```python
from build123d import *

# Parameters (mm, degrees)
SKETCH1_W                = 20
SKETCH1_H                = 80
BOSS_EXTRUDE1_DEPTH      = 5
BOSS_EXTRUDE2_DEPTH      = 10
BOSS_EXTRUDE2_DEPTH_BACK = 5
SKETCH2_W                = 20
SKETCH2_H                = 10.2
SKETCH3_W                = 20
SKETCH3_H                = 4.2
CUT_EXTRUDE1_DEPTH       = 10
BOSS_EXTRUDE3_DEPTH      = 194.158928137


with BuildPart() as part:
    # Sketch1 → Boss-Extrude1 (new body)
    with BuildSketch(Plane(origin=(0, 0, 0), x_dir=(1, 0, 0), z_dir=(0, 1, 0))):
        with Locations((10, 40)):
            Rectangle(SKETCH1_W, SKETCH1_H)
    extrude(amount=BOSS_EXTRUDE1_DEPTH)

    # Sketch2 → Boss-Extrude2 (add, two sides: drawn at the far end of the back side and taken through both)
    with BuildSketch(Plane.XZ.offset(-BOSS_EXTRUDE2_DEPTH_BACK)):
        with Locations((10, 5.1)):
            Rectangle(SKETCH2_W, SKETCH2_H)
    extrude(amount=BOSS_EXTRUDE2_DEPTH + BOSS_EXTRUDE2_DEPTH_BACK)

    # Sketch3 → Cut-Extrude1 (cut)
    with BuildSketch(Plane.XZ.offset(10)):
        with Locations((10, 5.1)):
            Rectangle(SKETCH3_W, SKETCH3_H)
    extrude(amount=-CUT_EXTRUDE1_DEPTH, mode=Mode.SUBTRACT)

    # Sketch5 → Boss-Extrude3 (add)
    with BuildSketch(Plane.ZY):
        Polygon((3, 0), (7.2, 0), (7.2, 5), (-80, 5), (-80, 0), (0, 0), (0, -10), (3, -10), align=None)
        Polygon((7.2, -10), (10.2, -10), (10.2, 5), (7.2, 5), (7.2, 0), align=None)
    extrude(amount=BOSS_EXTRUDE3_DEPTH)


solid = part.part
```
Geometry: final body of the model. Coordinates: model frame, mm. A direction names the side the tool comes from. Coordinates: 2 decimals unless noted, no trailing zeros. Write each loop counter-clockwise with the first axis right and the second up, starting at its lowest first coordinate (ties: lowest second). Pieces come first, ordered by that corner, then holes. Notation, with made-up numbers: M -23,-37.75 L -18,-37.75 A33 cw -18,1.25 Z; hole C -16,27 d1. An arc over 180 degrees is marked long. Answer as CSV lines item,"result". Start each with the question number.
Q1. Cut plane C-C on z = -67.5. Return the cut outline in (x, y).
Q2. Pin query (flat end, axial travel): P1, Ø5, axis at x = -136, y = -7, coming from the -Z side; P2, Ø5, axis at x = -148, z = -22, coming from the -Y side. Return the tip coordinate at first contact, or that it passes through.
Q3. Mould query, pull axis Z, two halves, no side actions, for faces 4 (the flat face through (20, 1, -28)), 5 (the flat face through (-86, -5, 0)), 6 (the flat face through (-86, -5, 7.2)). Classes: released by +Z, released by -Z, zero draft, split by the parting line, or undercut.
Q4. Line query: line 1 (Z direction, x = -131, y = -1); line 2 (Y direction, x = -11.5, z = -22). Output: solid intervals per line, ascending. Write a range as from..to.
Q5. Reachability of faces 1 (the flat face through (-194.159, 1, -28)), 2 (the flat face through (-86, 0, -41)), 3 (the flat face through (-86, 0, 5)) from +Z, -Z, +X, -X, +Y, -Y: full face, straight path, thin tool, end or side. Return the list, or none.
Q6. Cut plane A-A on y = -2.5. Return the cut outline in (x, z).
Q7. Cut plane B-B on x = -75. Return the cut outline in (y, z).
Findings below:
1,outline,"M -194.16,0 L 20,0 L 20,5 L -194.16,5 Z"
2,P1,"stops at z = 0"
2,P2,"stops at y = 0"
3,face 4,"zero draft"
3,face 5,"released by -Z"
3,face 6,"undercut"
4,line 1,"z = 0..3, 7.2..10.2"
4,line 2,"y = 0..5"
5,face 1,"+Z, -Z, -X, +Y, -Y"
5,face 2,"-Z, +X, -X, -Y"
5,face 3,"+X, -X, -Y"
6,outline,"M -194.16,0 L 20,0 L 20,3 L -194.16,3 Z; M -194.16,7.2 L 20,7.2 L 20,10.2 L -194.16,10.2 Z"
7,outline,"M -10,0 L 0,0 L 0,-80 L 5,-80 L 5,10.2 L -10,10.2 L -10,7.2 L 0,7.2 L 0,3 L -10,3 Z"
